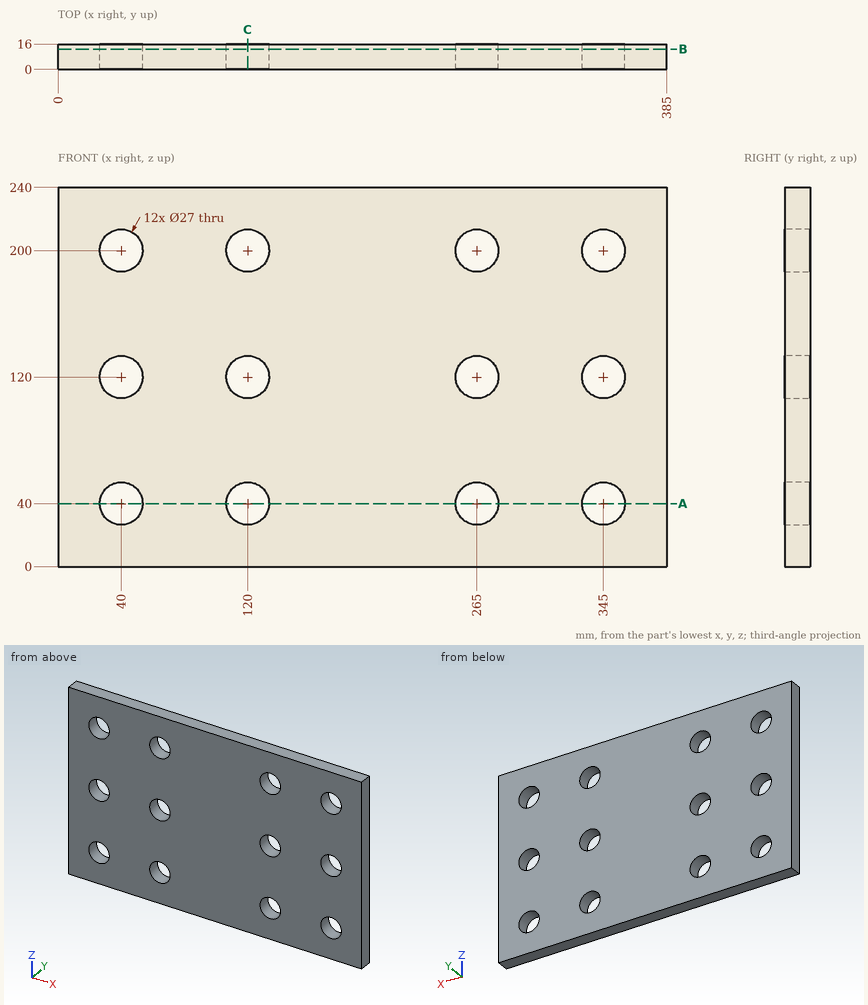
Here's the drawing with two shaded views (mm, measured from the low corner). I have some questions. Give positions to 0.01 mm unless a question says otherwise; leave off trailing zeros. Order: outer loops, then holes, each group sorted by start corner. A loop starts at its lowest first (then second) coordinate and runs counter-clockwise, first axis right, second up. Notation, with made-up numbers: (-13.5, 56) -> (-3.5, 56) arc R29 ccw to (-3.5, 80) -> close; hole circle Ø5 at (25.5, -39.75). An arc over 180 degrees is marked (long way). One line per item, written item: value. Start each with the question number.
1. Imagine slicing it at B-B, the plane y = 12.75. Count the separate pieces of the cut face and the enclosed holes in it, plus the area to 3 significant figures.
2. Imagine slicing it at A-A, the plane z = 40. List the corners of the cut face in (x, y) for me, plus the area to 3 significant figures.
3. Will this pin go through, and if not, where does the flat tip stop? pin 1 Ø21.5 at (x, z) = (265, 120) entering from -Y.
4. I need wall thicknesses on probe 1 along X at (y, z) = (9, 120); probe 2 along X at (y, z) = (12, 44); probe 3 along Z at (x, y) = (350.5, 11.75). Which ranges of each line are inside material? Lowest first, please. Write a range as from..to.
5. Imagine slicing it at C-C, the plane x = 120. List the corners of the cut face in (y, z) for me.
Values follow:
1. separate pieces: 1
1. enclosed holes: 12
1. area: 85,500 mm2
2. outline: (0, 0) -> (26.5, 0) -> (26.5, 16) -> (0, 16) -> close; (53.5, 0) -> (106.5, 0) -> (106.5, 16) -> (53.5, 16) -> close; (133.5, 0) -> (251.5, 0) -> (251.5, 16) -> (133.5, 16) -> close; (278.5, 0) -> (331.5, 0) -> (331.5, 16) -> (278.5, 16) -> close; (358.5, 0) -> (385, 0) -> (385, 16) -> (358.5, 16) -> close
2. area: 4,430 mm2
3. pin 1: passes through
4. probe 1: x = 0..26.5, 53.5..106.5, 133.5..251.5, 278.5..331.5, 358.5..385
4. probe 2: x = 0..27.11, 52.89..107.11, 132.89..252.11, 277.89..332.11, 357.89..385
4. probe 3: z = 0..27.67, 52.33..107.67, 132.33..187.67, 212.33..240
5. outline: (0, 0) -> (16, 0) -> (16, 26.5) -> (0, 26.5) -> close; (0, 53.5) -> (16, 53.5) -> (16, 106.5) -> (0, 106.5) -> close; (0, 133.5) -> (16, 133.5) -> (16, 186.5) -> (0, 186.5) -> close; (0, 213.5) -> (16, 213.5) -> (16, 240) -> (0, 240) -> close
